Geometry check sheet. Reference: the model listing, model coordinates, mm. A direction names the side the tool comes from. Round coordinates to 2 decimals unless told otherwise and drop trailing zeros. Write each loop counter-clockwise with the first axis right and the second up, starting at its lowest first coordinate (ties: lowest second). Pieces come first, ordered by that corner, then holes.
Item 1: Depth check by flat-ended pin: P1, Ø1.5, axis at x = 80, z = 9, coming from the +Y side; P2, Ø3, axis at y = 3, z = 7, coming from the -X side; P3, Ø1.5, axis at x = 80.5, z = 7.5, coming from the -Y side; P4, Ø11.5, axis at x = 97, y = 0, coming from the -Z side. Enter the tip coordinate at first touch or a pass-through.
Item 2: Cross-section at A-A (y = 0). Enter the section's corners in (x, z), then the cut area to 3 significant figures.
Item 3: Cross-section at D-D (y = 13). Enter the section's corners in (x, z).
Item 4: Draft check along Y on faces 6 (the face through (91, 5, 10)), 7 (the face through (78, -6, 5)), 8 (the face through (85.5, 9.1, 10.5)). Enter one of: pulls with the +Y half, pulls with the -Y half, needs draft (parallel to the pull), parting line crosses it, or undercut.
Item 5: Cross-section at B-B (z = 1.5). Enter the section's corners in (x, y), then the cut area to 3 significant figures.
Item 6: Cross-section at C-C (x = 97). Enter the section's corners in (y, z), then the cut area to 3 significant figures.
Item 7: Scan lines: probe 1 along Y at (x, z) = (97, 10.6); probe 2 along X at (y, z) = (0, 10.45); probe 3 along Y at (x, z) = (86.5, 8). Record each from-to range of solid material in increasing order.
Item 8: Access from +Z, -Z, +X, -X, +Y, -Y to the whole of each face (thin tool, end or side, straight path). Record for faces 1 (the face through (108.86, -1.82, 5.42)), 2 (the face through (89.5, 12, 5)), 3 (the face through (85.5, -4.2, 10.5)), 4 (the face through (107.1, 0.1, 4.9)), 5 (the face through (88.5, 10, 5)).
from build123d import *

# Parameters (mm, degrees)
CYLINDER040_R     = 6.5
CYLINDER040_DEPTH = 11
CYLINDER026_R     = 2.5
CYLINDER026_DEPTH = 11
CYLINDER025_R     = 2.5
CYLINDER025_DEPTH = 11
BOX006_W          = 1
BOX006_H          = 7
BOX006_DEPTH      = 11
BOX_W             = 3
BOX_H             = 20
BOX_DEPTH         = 1
CYLINDER024_R     = 12
CYLINDER024_DEPTH = 1
PAD011_DEPTH      = 10
BOX005_W          = 177
BOX005_H          = 100
BOX005_DEPTH      = 10
CYLINDER018_R     = 7.5
CYLINDER018_DEPTH = 10
CYLINDER016_R     = 10
CYLINDER016_DEPTH = 10
CYLINDER017_R     = 7.5
CYLINDER017_DEPTH = 10
CYLINDER019_R     = 10
CYLINDER019_DEPTH = 10
PAD009_DEPTH      = 6.5
PAD008_DEPTH      = 4
PAD010_DEPTH      = 10
CYLINDER021_R     = 7.5
CYLINDER021_DEPTH = 10
CYLINDER020_R     = 10
CYLINDER020_DEPTH = 10
CYLINDER022_R     = 7.5
CYLINDER022_DEPTH = 10
CYLINDER023_R     = 10
CYLINDER023_DEPTH = 10
TUBE_R            = 12
TUBE_R_2          = 10.1
TUBE_DEPTH        = 10
BOX007_W          = 19
BOX007_H          = 1
BOX007_DEPTH      = 11


with BuildPart() as cilindro040:
    # Cylinder040 → Cylinder040 (new body)
    with BuildSketch(Plane(origin=(-97, 0, 0), x_dir=(1, 0, 0), z_dir=(0, 0, 1))):
        Circle(CYLINDER040_R)
    extrude(amount=CYLINDER040_DEPTH)


with BuildPart() as cilindro026:
    # Cylinder026 → Cylinder026 (new body)
    with BuildSketch(Plane(origin=(-83, 10, 0), x_dir=(1, 0, 0), z_dir=(0, 0, 1))):
        Circle(CYLINDER026_R)
    extrude(amount=CYLINDER026_DEPTH)


with BuildPart() as cilindro025:
    # Cylinder025 → Cylinder025 (new body)
    with BuildSketch(Plane(origin=(-75, 0, 0), x_dir=(1, 0, 0), z_dir=(0, 0, 1))):
        Circle(CYLINDER025_R)
    extrude(amount=CYLINDER025_DEPTH)


with BuildPart() as cubo002:
    # Box006 → Box006 (new body)
    with BuildSketch(Plane(origin=(-89.5, 8, 0), x_dir=(1, 0, 0), z_dir=(0, 0, 1))):
        with Locations((0.5, 3.5)):
            Rectangle(BOX006_W, BOX006_H)
    extrude(amount=BOX006_DEPTH)


with BuildPart() as cubo001:
    # Box → Box (new body)
    with BuildSketch(Plane(origin=(-88.5, -5, 10), x_dir=(1, 0, 0), z_dir=(0, 0, 1))):
        with Locations((1.5, 10)):
            Rectangle(BOX_W, BOX_H)
    extrude(amount=BOX_DEPTH)


with BuildPart() as cilindro024:
    # Cylinder024 → Cylinder024 (new body)
    with BuildSketch(Plane(origin=(-97, 0, 10), x_dir=(1, 0, 0), z_dir=(0, 0, 1))):
        Circle(CYLINDER024_R)
    extrude(amount=CYLINDER024_DEPTH)


with BuildPart() as body008:
    # Sketch011 → Pad011 (new body)
    with BuildSketch(Plane.XY):
        Polygon((8.5, 4.907477), (0, 9.814955), (-8.5, 4.907477), (-8.5, -4.907477), (0, -9.814955), (8.5, -4.907477), align=None)
    extrude(amount=PAD011_DEPTH)


with BuildPart() as body008_1:
    # Body008 placement: moved
    add(body008.part.moved(Location((0, 45.1, 0))))


with BuildPart() as cut018:
    # Box005 → Box005 (new body)
    with BuildSketch(Plane(origin=(-88.5, -5, 0), x_dir=(1, 0, 0), z_dir=(0, 0, 1))):
        with Locations((88.5, 50)):
            Rectangle(BOX005_W, BOX005_H)
    extrude(amount=BOX005_DEPTH)

    # Cut018: cut Body008
    add(body008_1.part, mode=Mode.SUBTRACT)


with BuildPart() as cilindro018:
    # Cylinder018 → Cylinder018 (new body)
    with BuildSketch(Plane(origin=(0, 20, 0), x_dir=(1, 0, 0), z_dir=(0, 0, 1))):
        Circle(CYLINDER018_R)
    extrude(amount=CYLINDER018_DEPTH)


with BuildPart() as obj1:
    # Cylinder016 → Cylinder016 (new body)
    with BuildSketch(Plane(origin=(0, 20, 0), x_dir=(1, 0, 0), z_dir=(0, 0, 1))):
        Circle(CYLINDER016_R)
    extrude(amount=CYLINDER016_DEPTH)

    # Cut014: cut Cilindro018
    add(cilindro018.part, mode=Mode.SUBTRACT)


with BuildPart() as obj1_1:
    # Cut014 placement: moved
    add(obj1.part.moved(Location((-97, -20, 0))))


with BuildPart() as cilindro017:
    # Cylinder017 → Cylinder017 (new body)
    with BuildSketch(Plane(origin=(0, 20, 0), x_dir=(1, 0, 0), z_dir=(0, 0, 1))):
        Circle(CYLINDER017_R)
    extrude(amount=CYLINDER017_DEPTH)


with BuildPart() as fusion007:
    # Cylinder019 → Cylinder019 (new body)
    with BuildSketch(Plane(origin=(0, 20, 0), x_dir=(1, 0, 0), z_dir=(0, 0, 1))):
        Circle(CYLINDER019_R)
    extrude(amount=CYLINDER019_DEPTH)

    # Cut015: cut Cilindro017
    add(cilindro017.part, mode=Mode.SUBTRACT)


with BuildPart() as fusion007_1:
    # Cut015 placement: moved
    add(fusion007.part.moved(Location((97, -20, 0))))

    # Fusion007: union obj1
    add(obj1_1.part)


with BuildPart() as cuerpo005:
    # Sketch010 → Pad009 (new body)
    with BuildSketch(Plane.XY):
        Polygon((0, 7.505553), (-6.5, 3.752777), (-6.5, -3.752777), (0, -7.505553), (6.5, -3.752777), (6.5, 3.752777), align=None)
    extrude(amount=PAD009_DEPTH)

    # Sketch009 (on Face8 of Pad009) → Pad008 (join)
    with BuildSketch(Plane.XY.offset(6.5)):
        Polygon((0, 5.773503), (-5, 2.886751), (-5, -2.886751), (0, -5.773503), (5, -2.886751), (5, 2.886751), align=None)
    extrude(amount=PAD008_DEPTH)


with BuildPart() as cut016:
    # Sketch008 → Pad010 (new body)
    with BuildSketch(Plane.XY):
        Polygon((0, 9.814955), (-8.5, 4.907477), (-8.5, -4.907477), (0, -9.814955), (8.5, -4.907477), (8.5, 4.907477), align=None)
    extrude(amount=PAD010_DEPTH)

    # Cut016: cut Cuerpo005
    add(cuerpo005.part, mode=Mode.SUBTRACT)


with BuildPart() as cut016_1:
    # Cut016 placement: moved
    add(cut016.part.moved(Location((0, 45.1, 0))))


with BuildPart() as cilindro021:
    # Cylinder021 → Cylinder021 (new body)
    with BuildSketch(Plane(origin=(0, 20, 0), x_dir=(1, 0, 0), z_dir=(0, 0, 1))):
        Circle(CYLINDER021_R)
    extrude(amount=CYLINDER021_DEPTH)


with BuildPart() as obj2:
    # Cylinder020 → Cylinder020 (new body)
    with BuildSketch(Plane(origin=(0, 20, 0), x_dir=(1, 0, 0), z_dir=(0, 0, 1))):
        Circle(CYLINDER020_R)
    extrude(amount=CYLINDER020_DEPTH)

    # Cut017: cut Cilindro021
    add(cilindro021.part, mode=Mode.SUBTRACT)


with BuildPart() as obj2_1:
    # Cut017 placement: moved
    add(obj2.part.moved(Location((-97, -20, 0))))


with BuildPart() as cilindro022:
    # Cylinder022 → Cylinder022 (new body)
    with BuildSketch(Plane(origin=(0, 20, 0), x_dir=(1, 0, 0), z_dir=(0, 0, 1))):
        Circle(CYLINDER022_R)
    extrude(amount=CYLINDER022_DEPTH)


with BuildPart() as fusion008:
    # Cylinder023 → Cylinder023 (new body)
    with BuildSketch(Plane(origin=(0, 20, 0), x_dir=(1, 0, 0), z_dir=(0, 0, 1))):
        Circle(CYLINDER023_R)
    extrude(amount=CYLINDER023_DEPTH)

    # Cut019: cut Cilindro022
    add(cilindro022.part, mode=Mode.SUBTRACT)


with BuildPart() as fusion008_1:
    # Cut019 placement: moved
    add(fusion008.part.moved(Location((97, -20, 0))))

    # Fusion009: union obj2
    add(obj2_1.part)


with BuildPart() as fusion008_2:
    # Fusion009 placement: moved
    add(fusion008_1.part.moved(Location((0, 90, 0))))

    # Fusion008: union Cut018, Fusion007, Cut016
    add(cut018.part)
    add(fusion007_1.part)
    add(cut016_1.part)


with BuildPart() as cut020:
    # Tube → Tube (new body)
    with BuildSketch(Plane(origin=(-97, 0, 0), x_dir=(1, 0, 0), z_dir=(0, 0, 1))):
        Circle(TUBE_R)
        Circle(TUBE_R_2, mode=Mode.SUBTRACT)
    extrude(amount=TUBE_DEPTH)

    # Cut020: cut Fusion008
    add(fusion008_2.part, mode=Mode.SUBTRACT)


with BuildPart() as cut034:
    # Box007 → Box007 (new body)
    with BuildSketch(Plane(origin=(-87.5, -6, 0), x_dir=(1, 0, 0), z_dir=(0, 0, 1))):
        with Locations((9.5, 0.5)):
            Rectangle(BOX007_W, BOX007_H)
    extrude(amount=BOX007_DEPTH)

    # Fusion010: union Cubo002, Cubo001, Cilindro024, Cut020
    add(cubo002.part)
    add(cubo001.part)
    add(cilindro024.part)
    add(cut020.part)

    # Cut021: cut Cilindro025
    add(cilindro025.part, mode=Mode.SUBTRACT)

    # Cut022: cut Cilindro026
    add(cilindro026.part, mode=Mode.SUBTRACT)

    # Cut034: cut Cilindro040
    add(cilindro040.part, mode=Mode.SUBTRACT)


with BuildPart() as part_mirroring:
    # Part__Mirroring: instance of Cut034
    add(cut034.part.mirror(Plane(origin=(0, 0, 0), x_dir=(0, -1, 0), z_dir=(1, 0, 0))))


solid = part_mirroring.part
Resolved:
1. P1: stops at y = -5
1. P2: stops at x = 106.04
1. P3: stops at y = -6
1. P4: passes through
2. outline: (85, 10) - (90.5, 10) - (90.5, 11) - (85, 11) - close; (103.5, 10) - (107.1, 10) - (107.1, 0) - (109, 0) - (109, 11) - (103.5, 11) - close
2. area: 30.0 mm2
3. outline: (85.5, 10) - (88.5, 10) - (88.5, 0) - (89.5, 0) - (89.5, 11) - (85.5, 11) - close
4. face 6: undercut
4. face 7: pulls with the -Y half
4. face 8: needs draft
5. outline: (68.5, -6) - (86.61, -6) arc R12 ccw (long way) to (89.5, 9.37) - (89.5, 15) - (88.5, 15) - (88.5, 5.46) arc R10.1 cw (long way) to (88.22, -5) - (68.5, -5) - close
5. area: 131 mm2
6. outline: (-12, 0) - (-10.1, 0) - (-10.1, 10) - (-6.5, 10) - (-6.5, 11) - (-12, 11) - close; (6.5, 10) - (10.1, 10) - (10.1, 0) - (12, 0) - (12, 11) - (6.5, 11) - close
6. area: 49.0 mm2
7. probe 1: y = -12 to -6.5, 6.5 to 12
7. probe 2: x = 85 to 90.5, 103.5 to 109
7. probe 3: y = -6 to -5
8. face 1: +Z, -Z
8. face 2: +Z, -Z, +Y
8. face 3: +Z, -Z, -X
8. face 4: -Z
8. face 5: -Z, -X, +Y
